For this review, take the finished solid that the model builds, in its own axes (mm). A direction names the side the tool comes from. Coordinates: 2 decimals unless noted, no trailing zeros. Loops run counter-clockwise (first coordinate to the right, second up) from the corner with the lowest first, then second, coordinate; pieces in that order, holes last. Notation, with made-up numbers: M -38.75,51 L 17.25,51 A14 cw 17.25,77 Z; hole C 58.5,39.5 d5. An arc over 180 degrees is marked long. Answer as a JSON object with one key per item and string values. Group by question number.
Item 1: Add section D-D (x = -21). State the section outline as (y, z) points, then the cut area to 3 significant figures.
Item 2: Add section C-C (z = 4.75). State the section outline as (x, y) points, then the cut area to 3 significant figures.
Item 3: Add section A-A (y = 0). State the section outline as (x, z) points, then the cut area to 3 significant figures.
Item 4: Add section B-B (x = 27). State the section outline as (y, z) points, then the cut area to 3 significant figures.
Item 5: Insertion check: pin 1 (5 mm diameter, centred on x = -20, z = 1, fed in from +Y); pin 2 (1.2 mm diameter, centred on x = -35.5, y = 1, fed in from +Z); pin 3 (3 mm diameter, centred on x = 0, y = 0, fed in from -Z). Each pin has a flat end and moves straight along its axis. Give the tip position at first contact, or say it passes through.
Item 6: Mouldability with a two-part tool opening along Y and no side actions: class faces 1 (the face through (20.765, -39.923, 4.437)), 2 (the face through (35.293, -23.41, 8.014)), 3 (the face through (-1, 1, 9)) as +Y half, -Y half, draft (parallel to the pull), parting line (faces both ways), or undercut.
Item 7: Wall thickness on L1, parallel to Y at x = 0, z = 8; L2, parallel to Y at x = 13, z = 7.5; L3, parallel to X at y = -1, z = 3: over which ranges is each line inside the solid? List them lowest first. Write a range as from..to.
Item 8: Tool access review of faces 4 (the face through (-1, -9, 0)), 5 (the face through (13.503, 37.248, 8.014)), 6 (the face through (0, 0, 2)): name each direction out of +Z, -Z, +X, -X, +Y, -Y from which nothing blocks a thin tool from reaching the whole face with its end or side.
from build123d import *

# Parameters (mm, degrees)
F0_R     = 45
F0_R_2   = 2
F1_DEPTH = 9
F2_DEPTH = 2
F3_R     = 2
F4_DEPTH = 2


with BuildPart() as f1:
    # F0 (on Top) → F1 (new body)
    with BuildSketch(Plane.XY):
        Circle(F0_R)
        Circle(F0_R_2, mode=Mode.SUBTRACT)
        Circle(F0_R_2)
    extrude(amount=F1_DEPTH)

    # F0 (on Top) → F2 (cut)
    with BuildSketch(Plane.XY):
        Circle(F0_R_2)
    extrude(amount=F2_DEPTH, mode=Mode.SUBTRACT)

    # F3 (on face) → F4 (cut)
    with BuildSketch(Plane.XY.offset(9)):
        with Locations((-36.051724, 0)):
            Circle(F3_R)
        with Locations((12.580568, 39.022164)):
            Circle(F3_R)
        with Locations((33.445747, -22.644383)):
            Circle(F3_R)
    extrude(amount=-F4_DEPTH, mode=Mode.SUBTRACT)


solid = f1.part
From the geometry:
{
 "1": {"outline": "M -39.8,0 L 39.8,0 L 39.8,9 L -39.8,9 Z", "area": "716 mm²"},
 "2": {"outline": "C 0,0 d90", "area": "6,360 mm²"},
 "3": {"outline": "M -45,0 L -2,0 L -2,2 L 2,2 L 2,0 L 45,0 L 45,9 L -34.05,9 L -34.05,7 L -38.05,7 L -38.05,9 L -45,9 Z", "area": "794 mm²"},
 "4": {"outline": "M -36,0 L 36,0 L 36,9 L -36,9 Z", "area": "648 mm²"},
 "5": {"pin 1": "stops at y = 41.46", "pin 2": "stops at z = 7", "pin 3": "stops at z = 2"},
 "6": {"face 1": "parting line", "face 2": "undercut", "face 3": "draft"},
 "7": {"L1": "y = -45..45", "L2": "y = -43.08..37.07, 40.98..43.08", "L3": "x = -44.99..44.99"},
 "8": {"face 4": "-Z, +X, -X, +Y, -Y", "face 5": "+Z", "face 6": "-Z"}
}
